from build123d import *

# Parameters (mm, degrees)
F0_R      = 1.3335
F1_DEPTH  = 6.35
F2_W      = 16.51
F2_H      = 4.318
F3_DEPTH  = 6.351
F5_DEPTH  = 1.778
F6_DEPTH  = 6.604
F7_DEPTH  = 3.429
F4_W      = 15.748
F4_H      = 52.5018
F8_DEPTH  = 2.54
F9_W      = 6.35
F9_H      = 6.35
F10_W     = 6.35
F10_H     = 6.35
F11_DEPTH = 2.54
F12_W     = 6.35
F12_H     = 2.54
F13_DEPTH = 14.605
F14_W     = 3.175
F14_H     = 2.54
F15_DEPTH = 20.956
F16_W     = 1.27
F16_H     = 14.605
F17_W     = 1.27
F17_H     = 14.605
F18_DEPTH = 3.175


with BuildPart() as f1:
    # F0 (on Top) → F1 (new body)
    with BuildSketch(Plane.XY):
        with BuildLine():
            Line((58.42, 0), (0, 0))
            Line((0, 0), (0, -66.3448))
            Line((0, -66.3448), (14.9897452514, -66.3448))
            ThreePointArc((14.9897452514, -66.3448), (16.0999808785, -61.7704024843), (19.9771, -64.4398))
            ThreePointArc((19.9771, -64.4398), (19.7889975157, -65.4594191215), (19.2494547486, -66.3448))
            Line((19.2494547486, -66.3448), (39.1705452514, -66.3448))
            ThreePointArc((39.1705452514, -66.3448), (40.2807808785, -61.7704024843), (44.1579, -64.4398))
            ThreePointArc((44.1579, -64.4398), (43.9697975157, -65.4594191215), (43.4302547486, -66.3448))
            Line((43.4302547486, -66.3448), (58.42, -66.3448))
            Line((58.42, -66.3448), (58.42, 0))
        make_face()
        with Locations((17.1196, -2.2098)):
            Circle(F0_R, mode=Mode.SUBTRACT)
        with Locations((41.3004, -2.2098)):
            Circle(F0_R, mode=Mode.SUBTRACT)
        with BuildLine():
            ThreePointArc((19.9771, -64.4398), (16.0999808785, -61.7704024843), (14.9897452514, -66.3448))
            Line((14.9897452514, -66.3448), (19.2494547486, -66.3448))
            ThreePointArc((19.2494547486, -66.3448), (19.7889975157, -65.4594191215), (19.9771, -64.4398))
        make_face()
        with Locations((17.1196, -64.4398)):
            Circle(F0_R, mode=Mode.SUBTRACT)
        with BuildLine():
            Line((39.1705452514, -66.3448), (43.4302547486, -66.3448))
            ThreePointArc((43.4302547486, -66.3448), (43.9697975157, -65.4594191215), (44.1579, -64.4398))
            ThreePointArc((44.1579, -64.4398), (40.2807808785, -61.7704024843), (39.1705452514, -66.3448))
        make_face()
        with Locations((41.3004, -64.4398)):
            Circle(F0_R, mode=Mode.SUBTRACT)
    extrude(amount=F1_DEPTH)

    # F2 (on face) → F3 (cut, through all)
    with BuildSketch(Plane.XY.offset(6.35)):
        with Locations((29.21, -2.159)):
            Rectangle(F2_W, F2_H)
    extrude(amount=-F3_DEPTH, mode=Mode.SUBTRACT)

    # F5 (add): a face of the model
    f5_faces = [f1.faces().sort_by_distance(p)[0] for p in [
        (29.21, -66.3448, 3.175),
    ]]
    extrude(f5_faces, amount=F5_DEPTH)

    # F0 (on Top) → F6 (join)
    with BuildSketch(Plane.XY):
        with BuildLine():
            Line((39.1705452514, -66.3448), (43.4302547486, -66.3448))
            ThreePointArc((43.4302547486, -66.3448), (43.9697975157, -65.4594191215), (44.1579, -64.4398))
            ThreePointArc((44.1579, -64.4398), (40.2807808785, -61.7704024843), (39.1705452514, -66.3448))
        make_face()
        with Locations((41.3004, -64.4398)):
            Circle(F0_R, mode=Mode.SUBTRACT)
        with BuildLine():
            ThreePointArc((19.9771, -64.4398), (16.0999808785, -61.7704024843), (14.9897452514, -66.3448))
            Line((14.9897452514, -66.3448), (19.2494547486, -66.3448))
            ThreePointArc((19.2494547486, -66.3448), (19.7889975157, -65.4594191215), (19.9771, -64.4398))
        make_face()
        with Locations((17.1196, -64.4398)):
            Circle(F0_R, mode=Mode.SUBTRACT)
        with BuildLine():
            Line((19.2494547486, -66.3448), (14.9897452514, -66.3448))
            ThreePointArc((14.9897452514, -66.3448), (17.1196, -67.2973), (19.2494547486, -66.3448))
        make_face()
        with BuildLine():
            ThreePointArc((39.1705452514, -66.3448), (41.3004, -67.2973), (43.4302547486, -66.3448))
            Line((43.4302547486, -66.3448), (39.1705452514, -66.3448))
        make_face()
    extrude(amount=F6_DEPTH)

    # F7 (cut): faces of the model
    f7_faces = [f1.faces().sort_by_distance(p)[0] for p in [
        (19.1892133591, -62.5886815367, 6.604),
        (43.3700133591, -62.5886815367, 6.604),
    ]]
    extrude(f7_faces, amount=-F7_DEPTH, mode=Mode.SUBTRACT)

    # F4 (on face) → F8 (join)
    with BuildSketch(Plane.XY.offset(6.35)):
        with Locations((29.21, -35.7759)):
            Rectangle(F4_W, F4_H)
    extrude(amount=F8_DEPTH)

    # F9 (on face) + F10 (on face) → F11 (join)
    with BuildSketch(Plane(origin=(0, 0, 0), x_dir=(-1, 0, 0), z_dir=(0, 1, 0))):
        with Locations((-17.78, 3.175)):
            Rectangle(F9_W, F9_H)
    with BuildSketch(Plane(origin=(0, 0, 0), x_dir=(-1, 0, 0), z_dir=(0, 1, 0))):
        with Locations((-40.64, 3.175)):
            Rectangle(F10_W, F10_H)
    extrude(amount=F11_DEPTH)

    # F12 (on face) → F13 (join)
    with BuildSketch(Plane.XY.offset(6.35)):
        with Locations((17.78, 1.27)):
            Rectangle(F12_W, F12_H)
        with Locations((40.64, 1.27)):
            Rectangle(F12_W, F12_H)
    extrude(amount=F13_DEPTH)

    # F14 (on face) → F15 (cut, through all)
    with BuildSketch(Plane(origin=(0, 0, 0), x_dir=(1, 0, 0), z_dir=(0, 0, -1))):
        with Locations((19.3675, -1.27)):
            Rectangle(F14_W, F14_H)
        with Locations((39.0525, -1.27)):
            Rectangle(F14_W, F14_H)
    extrude(amount=-F15_DEPTH, mode=Mode.SUBTRACT)

    # F16 (on face) + F17 (on face) → F18 (join)
    with BuildSketch(Plane(origin=(0, 2.54, 0), x_dir=(-1, 0, 0), z_dir=(0, 1, 0))):
        with Locations((-43.18, 13.6525)):
            Rectangle(F16_W, F16_H)
    with BuildSketch(Plane(origin=(0, 2.54, 0), x_dir=(-1, 0, 0), z_dir=(0, 1, 0))):
        with Locations((-15.24, 13.6525)):
            Rectangle(F17_W, F17_H)
    extrude(amount=F18_DEPTH)


solid = f1.part
Here's how the part is built. I have some questions about the finished solid (model axes, mm). A direction names the side the tool comes from. Give positions to 0.01 mm unless a question says otherwise; leave off trailing zeros. Loops run counter-clockwise (first coordinate to the right, second up) from the corner with the lowest first, then second, coordinate; pieces in that order, holes last. Notation, with made-up numbers: (88, -15) -> (147, -15) arc R32 cw to (147, 16) -> close; hole circle Ø4 at (16, 59.25). An arc over 180 degrees is marked (long way). One line per item, written item: value.
Q1. Suppose I cut it at A-A on z = 10.75. Please give me the cut outline in (x, y) (3 decimals).
Answers follow:
outline: (14.605, 0) -> (17.78, 0) -> (17.78, 2.54) -> (15.875, 2.54) -> (15.875, 5.715) -> (14.605, 5.715) -> close; (40.64, 0) -> (43.815, 0) -> (43.815, 5.715) -> (42.545, 5.715) -> (42.545, 2.54) -> (40.64, 2.54) -> close
Q2. If I drill on line 1 along X through (y, z) = (3.5, 18) (3 decimals); line 2 along Y through (x, z) = (18, 1.5); line 3 along Y through (x, z) = (19, 5.75), over which ranges is the centre line in solid material (lowest first)?
Answers follow:
line 1: 14.605 to 15.875, 42.545 to 43.815
line 2: -68.12 to -65.44, -63.44 to -3.21, -1.21 to 0
line 3: -68.12 to -66.59, -62.29 to 0
Q3. Suppose I cut it at B-B on y = -11. Please give me the cut outline in (x, z), then the cut area to 3 significant figures.
Answers follow:
outline: (0, 0) -> (58.42, 0) -> (58.42, 6.35) -> (37.08, 6.35) -> (37.08, 8.89) -> (21.34, 8.89) -> (21.34, 6.35) -> (0, 6.35) -> close
area: 411 mm^2
Q4. On a 3-axis mill with a long thin cutter (end or side, diameter ignored), from which of +Z, -Z, +X, -X, +Y, -Y can I reach the whole of each face in a straight line? I mean faces 5 (the face through (42.545, 4, 14)), 6 (the face through (41.92, -65.62, 1.57)), 7 (the face through (29, -9.525, 8)), 8 (the face through (42, -66, 3.175)), 9 (the face through (16, 0, 14)). Say none if no direction works.
Answers follow:
face 5: +Z, -Z, +Y
face 6: +Z, -Z
face 7: +Z, +X, -X, +Y
face 8: +Z
face 9: +Z, +X, -X, -Y
Q5. I'm going to push flat-ended pins straight in: pin 1 Ø3 at (y, z) = (2, 8) entering from -X (3 decimals); pin 2 Ø4.5 at (x, y) = (41, -66) entering from +Z; pin 3 Ø2 at (x, z) = (40.5, 16) entering from -Y; pin 4 Ø8 at (x, z) = (49, 12) entering from +Y. Where does each tip first touch, or does it pass through?
Answers follow:
pin 1: x = 14.605
pin 2: z = 6.35
pin 3: y = 0
pin 4: through
Q6. We'd pull the mould along X, two halves only. Please class faces 1 (the face through (20.955, -2, 3)), 2 (the face through (17, 2.54, 8)), 3 (the face through (42, 0, 14)), 4 (the face through (43.815, 3, 13)): pulls with the +X half, pulls with the -X half, needs draft (parallel to the pull), parting line crosses it, or undercut.
Answers follow:
face 1: undercut
face 2: undercut
face 3: needs draft
face 4: pulls with the +X half
Q7. Suppose I cut it at D-D on x = 25.5. Please give me the cut outline in (y, z) (3 decimals).
Answers follow:
outline: (-68.123, 0) -> (-4.318, 0) -> (-4.318, 6.35) -> (-9.525, 6.35) -> (-9.525, 8.89) -> (-62.027, 8.89) -> (-62.027, 6.35) -> (-68.123, 6.35) -> close
Q8. Suppose I cut it at C-C on x = 41.5. Please give me the cut outline in (y, z) (3 decimals).
Answers follow:
outline: (-68.123, 0) -> (-65.758, 0) -> (-65.758, 3.175) -> (-67.29, 3.175) -> (-67.29, 6.35) -> (-68.123, 6.35) -> close; (-63.121, 0) -> (-3.528, 0) -> (-3.528, 6.35) -> (-61.589, 6.35) -> (-61.589, 3.175) -> (-63.121, 3.175) -> close; (-0.891, 0) -> (2.54, 0) -> (2.54, 20.955) -> (0, 20.955) -> (0, 6.35) -> (-0.891, 6.35) -> close
